```python
from build123d import *

# Parameters (mm, degrees)
BOSS_EXTRUDE1_DEPTH = 5
SKETCH2_R           = 2
CUT_EXTRUDE1_DEPTH  = 5
SKETCH5_W           = 10
SKETCH5_H           = 5
CUT_EXTRUDE2_DEPTH  = 5
SKETCH6_R           = 2
BOSS_EXTRUDE4_DEPTH = 3


with BuildPart() as part:
    # Sketch1 → Boss-Extrude1 (new body)
    # profile 1 of 9: a face of its own
    with BuildSketch(Plane(origin=(0, 0, 0), x_dir=(1, 0, 0), z_dir=(0, 1, 0))):
        with BuildLine():
            ThreePointArc((4.898979486, -2.5), (5.347634392, -1.285615189), (5.5, 0))
            ThreePointArc((5.5, 0), (0, 5.5), (-5.5, 0))
            ThreePointArc((-5.5, 0), (-5.347634392, -1.285615189), (-4.898979486, -2.5))
            Line((-4.898979486, -2.5), (0, -2.5))
            Line((0, -2.5), (4.898979486, -2.5))
        make_face()
        with BuildLine():
            ThreePointArc((2.5, 0), (1.767766953, -1.767766953), (0, -2.5))
            ThreePointArc((0, -2.5), (-1.767766953, 1.767766953), (2.5, 0))
        make_face(mode=Mode.SUBTRACT)
    # profile 2 of 9: a face of its own
    with BuildSketch(Plane(origin=(0, 0, 0), x_dir=(1, 0, 0), z_dir=(0, 1, 0))):
        with BuildLine():
            ThreePointArc((0, -5.5), (2.872281323, -4.69041576), (4.898979486, -2.5))
            Line((4.898979486, -2.5), (0, -2.5))
            Line((0, -2.5), (0, -5.5))
        make_face()
    # profile 3 of 9: a face of its own
    with BuildSketch(Plane(origin=(0, 0, 0), x_dir=(1, 0, 0), z_dir=(0, 1, 0))):
        with BuildLine():
            Line((0, -2.5), (-4.898979486, -2.5))
            ThreePointArc((-4.898979486, -2.5), (-2.872281323, -4.69041576), (0, -5.5))
            Line((0, -5.5), (0, -2.5))
        make_face()
    # profile 4 of 9: a face of its own
    with BuildSketch(Plane(origin=(0, 0, 0), x_dir=(1, 0, 0), z_dir=(0, 1, 0))):
        with BuildLine():
            Line((25.742031851, -2.5), (11.729658022, -2.5))
            Line((11.729658022, -2.5), (4.898979486, -2.5))
            ThreePointArc((4.898979486, -2.5), (2.872281323, -4.69041576), (0, -5.5))
            Line((0, -5.5), (25.742031851, -5.5))
            Line((25.742031851, -5.5), (25.742031851, -2.5))
        make_face()
    # profile 5 of 9: a face of its own
    with BuildSketch(Plane(origin=(0, 0, 0), x_dir=(1, 0, 0), z_dir=(0, 1, 0))):
        with BuildLine():
            Line((11.729658022, -2.5), (5.5, 0))
            ThreePointArc((5.5, 0), (5.347634392, -1.285615189), (4.898979486, -2.5))
            Line((4.898979486, -2.5), (11.729658022, -2.5))
        make_face()
    # profile 6 of 9: a face of its own
    with BuildSketch(Plane(origin=(0, 0, 0), x_dir=(1, 0, 0), z_dir=(0, 1, 0))):
        with BuildLine():
            ThreePointArc((0, -5.5), (2.872281323, -4.69041576), (4.898979486, -2.5))
            Line((4.898979486, -2.5), (0, -2.5))
            Line((0, -2.5), (0, -5.5))
        make_face()
    # profile 7 of 9: a face of its own
    with BuildSketch(Plane(origin=(0, 0, 0), x_dir=(1, 0, 0), z_dir=(0, 1, 0))):
        with BuildLine():
            Line((0, -2.5), (-4.898979486, -2.5))
            ThreePointArc((-4.898979486, -2.5), (-2.872281323, -4.69041576), (0, -5.5))
            Line((0, -5.5), (0, -2.5))
        make_face()
    # profile 8 of 9: a face of its own
    with BuildSketch(Plane(origin=(0, 0, 0), x_dir=(1, 0, 0), z_dir=(0, 1, 0))):
        with BuildLine():
            ThreePointArc((-4.898979486, -2.5), (-5.347634392, -1.285615189), (-5.5, 0))
            Line((-5.5, 0), (-11.729658022, -2.5))
            Line((-11.729658022, -2.5), (-4.898979486, -2.5))
        make_face()
    # profile 9 of 9: a face of its own
    with BuildSketch(Plane(origin=(0, 0, 0), x_dir=(1, 0, 0), z_dir=(0, 1, 0))):
        with BuildLine():
            Line((-4.898979486, -2.5), (-11.729658022, -2.5))
            Line((-11.729658022, -2.5), (-25.742031851, -2.5))
            Line((-25.742031851, -2.5), (-25.742031851, -5.5))
            Line((-25.742031851, -5.5), (0, -5.5))
            ThreePointArc((0, -5.5), (-2.872281323, -4.69041576), (-4.898979486, -2.5))
        make_face()
    extrude(amount=BOSS_EXTRUDE1_DEPTH)

    # Sketch2 → Cut-Extrude1 (cut)
    with BuildSketch(Plane(origin=(0, 0, 2.5), x_dir=(-1, 0, 0), z_dir=(0, 0, -1))):
        Polygon((-25.742031851, 0), (-21.729658022, 0), (-21.729658022, 2.5), (-21.729658022, 5), (-25.742031851, 5), align=None)
        Polygon((21.729658022, 2.5), (21.729658022, 0), (25.742031851, 0), (25.742031851, 5), (21.729658022, 5), align=None)
        with Locations((16.729658022, 2.5)):
            Circle(SKETCH2_R)
        with Locations((-16.729658022, 2.5)):
            Circle(SKETCH2_R)
    extrude(amount=-CUT_EXTRUDE1_DEPTH, mode=Mode.SUBTRACT)

    # Sketch5 → Cut-Extrude2 (cut)
    with BuildSketch(Plane(origin=(0, 0, 2.5), x_dir=(-1, 0, 0), z_dir=(0, 0, -1))):
        with Locations((-16.729658022, 2.5)):
            Rectangle(SKETCH5_W, SKETCH5_H)
        with Locations((16.729658022, 2.5)):
            Rectangle(SKETCH5_W, SKETCH5_H)
    extrude(amount=-CUT_EXTRUDE2_DEPTH, mode=Mode.SUBTRACT)

    # Sketch6 → Boss-Extrude4 (add)
    # profile 1 of 6: a face of its own
    with BuildSketch(Plane.XY.offset(5.5)):
        Polygon((11.729658022, 11), (0, 11), (0, 8), (0, 5), (11.729658022, 5), align=None)
        with Locations((5.864829011, 8)):
            Circle(SKETCH6_R, mode=Mode.SUBTRACT)
    # profile 2 of 6: a face of its own
    with BuildSketch(Plane.XY.offset(5.5)):
        Polygon((0, 0), (0, -3), (0, -6), (11.729658022, -6), (11.729658022, 0), align=None)
        with Locations((5.864829011, -3)):
            Circle(SKETCH6_R, mode=Mode.SUBTRACT)
    # profile 3 of 6: a face of its own
    with BuildSketch(Plane.XY.offset(5.5)):
        with BuildLine():
            Line((0, 5), (0, 8))
            Line((0, 8), (-3.864829011, 8))
            ThreePointArc((-3.864829011, 8), (-5.864829011, 6), (-7.864829011, 8))
            Line((-7.864829011, 8), (-11.729658022, 8))
            Line((-11.729658022, 8), (-11.729658022, 5))
            Line((-11.729658022, 5), (0, 5))
        make_face()
    # profile 4 of 6: a face of its own
    with BuildSketch(Plane.XY.offset(5.5)):
        with BuildLine():
            Line((0, 8), (0, 11))
            Line((0, 11), (-11.729658022, 11))
            Line((-11.729658022, 11), (-11.729658022, 8))
            Line((-11.729658022, 8), (-7.864829011, 8))
            ThreePointArc((-7.864829011, 8), (-5.864829011, 10), (-3.864829011, 8))
            Line((-3.864829011, 8), (0, 8))
        make_face()
    # profile 5 of 6: a face of its own
    with BuildSketch(Plane.XY.offset(5.5)):
        with BuildLine():
            ThreePointArc((-7.864829011, -3), (-5.864829011, -1), (-3.864829011, -3))
            Line((-3.864829011, -3), (0, -3))
            Line((0, -3), (0, 0))
            Line((0, 0), (-11.729658022, 0))
            Line((-11.729658022, 0), (-11.729658022, -3))
            Line((-11.729658022, -3), (-7.864829011, -3))
        make_face()
    # profile 6 of 6: a face of its own
    with BuildSketch(Plane.XY.offset(5.5)):
        with BuildLine():
            Line((0, -3), (-3.864829011, -3))
            ThreePointArc((-3.864829011, -3), (-5.864829011, -5), (-7.864829011, -3))
            Line((-7.864829011, -3), (-11.729658022, -3))
            Line((-11.729658022, -3), (-11.729658022, -6))
            Line((-11.729658022, -6), (0, -6))
            Line((0, -6), (0, -3))
        make_face()
    extrude(amount=-BOSS_EXTRUDE4_DEPTH)


solid = part.part
```
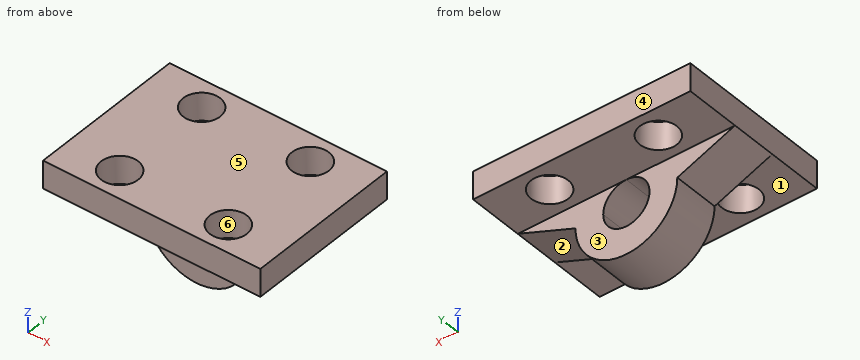
The listing builds one solid part. Answer for the finished solid, in the listing's coordinates (mm). Face numbers are marked on the shaded views. A direction names the side the tool comes from. Give positions to 0.01 mm unless a question says otherwise; leave off trailing zeros. Order: outer loops, then holes, each group sorted by start corner. A loop starts at its lowest first (then second) coordinate and runs counter-clockwise, first axis right, second up. Notation, with made-up numbers: (37, 28) - (56, 28) arc R19 cw to (56, 62) - close; hole circle Ø6 at (79.5, -18.5). An arc over 180 degrees is marked (long way). Answer in a Markdown table with one row per item. Add a question column.
Q1. The part is cut by section C-C (x = -1.5). Determine the outline of the cut face in (y, z).
Q2. The part is cut by section D-D (y = 2.5). Determine the outline of the cut face in (x, z).
Q3. The part is cut by section A-A (y = -1.5). Determine the outline of the cut face in (x, z).
Q4. Given P1, Ø1.5, axis at x = -2.5, y = 3.5, coming from the -Z side; P2, Ø4, axis at y = 2.5, z = 2, coming from the -X side; P3, Ø1.8, axis at x = -3, y = 8.5, coming from the -Z side; P4, Ø3, axis at x = 5.86, y = 8, coming from the -Z side, each flat-ended and moving along its own axis, determine where each tip first touches the part or whether it passes through.
Q5. Which of the six approach directions +Z, -Z, +X, -X, +Y, -Y give full straight-line access (tool end or side, diameter ignored) to the marked faces 1, 2 and 3?
Q6. For a pull along Y with two mould halves and no side action, classify the marked faces 4, 5 and 6 as released by +Y, released by -Y, zero draft, split by the parting line, or undercut.
Q7. Find the intervals of material crossed by line 1 along Y through (x, z) = (6, 3.5); line 2 along Z through (x, y) = (-10.5, 8.25); line 3 along Z through (x, y) = (0, 1.4), in increasing order. Write a range as [from, to].
Q8. The part is cut by section B-B (z = 1.5). Determine the outline of the cut face in (x, y).
Determined:
| question | item | result |
|---|---|---|
| 1 | outline | (-6, 2.5) - (0, 2.5) - (0, 2) - (5, 2) - (5, 2.5) - (11, 2.5) - (11, 5.5) - (-6, 5.5) - close; (0, -5.29) - (5, -5.29) - (5, -2) - (0, -2) - close |
| 2 | outline | (-11.73, 2.5) - (-5.5, 0) arc R5.5 ccw to (5.5, 0) - (11.73, 2.5) - (11.73, 5.5) - (-11.73, 5.5) - close; hole circle Ø5 at (0, 0) |
| 3 | outline | (-11.73, 2.5) - (-7.19, 2.5) - (-7.19, 5.5) - (-11.73, 5.5) - close; (-4.54, 2.5) - (4.54, 2.5) - (4.54, 5.5) - (-4.54, 5.5) - close; (7.19, 2.5) - (11.73, 2.5) - (11.73, 5.5) - (7.19, 5.5) - close |
| 4 | P1 | stops at z = -5.21 |
| 4 | P2 | stops at x = -11.73 |
| 4 | P3 | stops at z = 2.5 |
| 4 | P4 | passes through |
| 5 | face 1 | -Z, +X, -X, -Y |
| 5 | face 2 | -Z, +X, +Y, -Y |
| 5 | face 3 | -Z, +X, -X, +Y |
| 6 | face 4 | released by +Y |
| 6 | face 5 | zero draft |
| 6 | face 6 | undercut |
| 7 | line 1 | y = [-6, -5], [-1, 6], [10, 11] |
| 7 | line 2 | z = [2.5, 5.5] |
| 7 | line 3 | z = [-5.5, -2.5], [2.5, 5.5] |
| 8 | outline | (-9.24, 0) - (-2, 0) - (-2, 5) - (-9.24, 5) - close; (2, 0) - (9.24, 0) - (9.24, 5) - (2, 5) - close |
